Input: part model. Units: mm. Frame: model coordinates. Coordinates: 2 decimals unless noted, no trailing zeros. Order: outer loops, then holes, each group sorted by start corner. A loop starts at its lowest first (then second) coordinate and runs counter-clockwise, first axis right, second up.
Autodesk Inventor part; units mm, degrees
ref_plane "Start Plane" through (0, 0, -7.3433) normal (0, 0, 1) x (1, 0, 0)
ref_plane "End Plane" through (0, 0, 344.1675) normal (0, 0, 1) x (1, 0, 0)
ref_plane "Work Plane4" through (-6.6869, -8.3122, -7.3679) normal (0.3562, 0.4428, -0.8228) x (0.2838, -0.8903, -0.3562)
ref_plane "Start Plane" through (0, 0, -7.3433) normal (0, 0, 1) x (1, 0, 0)
ref_plane "End Plane" through (0, 0, 344.1675) normal (0, 0, 1) x (1, 0, 0)
sketch "Sketch" plane through (0, 0, 0) normal (0, 0, 1) x (1, 0, 0)
  circle A0 centre (0, 0) radius 6.9342
  circle A1 centre (0, 0) radius 10.668
  dimension "d0" = 21.336
  dimension "d1" = 3.7338
extrude "Body" add sketch "Sketch" along normal up to surface (351.5108 mm away) from surface at -7.3433
sketch "Sketch3" plane through (0, 0, 0) normal (0, 0, 1) x (1, 0, 0)
  line L0 (0, 0) -> (10, 0)
ref_plane "Work Plane3" through (0, 0, 0) normal (0, -1, 0) x (1, 0, 0)
sketch "Sketch4" plane through (0, 0, 0) normal (0, -1, 0) x (1, 0, 0)
  line L0 (-2, -7.3433) -> (12, -7.3433)
  line L1 (-2, 344.1675) -> (12, 344.1675)
  dimension "d7" = 351.5108
ref_plane "Work Plane4" through (-6.6869, -8.3122, -7.3679) normal (0.3562, 0.4428, -0.8228) x (0.2838, -0.8903, -0.3562)
split "Split1" plane through (-6.6869, -8.3122, -7.3679) removes the side toward (0.3562, 0.4428, -0.8228)
ref_plane "Work Plane5" through (6.3956, -8.5383, -22.5235) normal (-0.5418, 0.7233, -0.4281) x (0.4867, 0.6852, 0.5418)
split "Split2" plane through (6.3956, -8.5383, -22.5235) removes the side toward (-0.5418, 0.7233, -0.4281)
ref_plane "Work Plane6" through (-10.4471, 2.1596, -41.6241) normal (0.9486, -0.1961, -0.2483) x (-0.1971, 0.2475, -0.9486)
split "Split3" plane through (-10.4471, 2.1596, -41.6241) removes the side toward (0.9486, -0.1961, -0.2483)
ref_plane "Work Plane7" through (-0.5919, -10.6516, 344.93) normal (0.026, 0.467, 0.8839) x (0.9996, -0.0064, -0.026)
split "Split4" plane through (-0.5919, -10.6516, 344.93) removes the side toward (0.026, 0.467, 0.8839)
ref_plane "Work Plane8" through (-10.4471, 2.1596, 352.5336) normal (0.7628, -0.1577, 0.6272) x (0.6424, 0.0739, -0.7628)
split "Split5" plane through (-10.4471, 2.1596, 352.5336) removes the side toward (0.7628, -0.1577, 0.6272)
ref_plane "Work Plane9" through (6.3956, -8.5383, 369.7521) normal (-0.5658, 0.7554, 0.3305) x (0.7594, 0.3213, 0.5658)
split "Split6" plane through (6.3956, -8.5383, 369.7521) removes the side toward (-0.5658, 0.7554, 0.3305)
equation "\"d0\" = G_H"
equation "\"d1\" = G_T"
equation "\"d2\" = G_L"
equation "\"G_H\" = 21.336"
equation "\"G_T\" = 3.7338"
equation "\"G_L\" = 351.51084"
equation "\"G_OFFSET_START\" = 7.34335"
equation "\"G_OFFSET_END\" = 4.88279"
equation "\"d4\" = -G_OFFSET_START"
equation "\"d5\" = G_OFFSET_END + B_L"
equation "\"B_L\" = 339.28471"
properties part number "ANSI - 1/2 x 0.147 - 13.839" material "Steel, Mild"
Item 1: Draft query along X for faces 1 (the face through (5.735, -8.995, 165.952)), 2 (the face through (-0.903, -6.875, 166.412)), 3 (the face through (-6.44, 3.09, 13.37)). Return one class per face: pulls with the +X half, pulls with the -X half, needs draft (parallel to the pull), parting line crosses it, or undercut.
Response values:
face 1: parting line crosses it
face 2: undercut
face 3: pulls with the -X half
Item 2: Ray query, probe 1 along Y at (x, z) = (0, 224.5); probe 2 along X at (y, z) = (4.5, 117). Return the intervals inside material, ascending.
Response values:
probe 1: y = -10.67 to -6.93, 6.93 to 10.67
probe 2: x = -9.67 to -5.28, 5.28 to 9.67
Item 3: Cut plane C-C on z = 320. Return loops of the section in (x, y).
Response values:
outline: (-10.66, 0.46) arc R10.67 ccw (long way) to (2.56, 10.36) - (-2.79, 6.35) arc R6.93 cw (long way) to (-5.31, 4.46) - close
Item 4: Pin query (flat end, axial travel): pin 1 Ø1 at (x, y) = (7, -6.5) entering from +Z; pin 2 Ø1.5 at (y, z) = (-6.5, 48.5) entering from -X; pin 3 Ø10 at (y, z) = (-5, 270) entering from -X; pin 4 Ø8 at (x, y) = (-6.5, 3.5) entering from -Z. Return the tip coordinate at first contact, or that it passes through.
Response values:
pin 1: stops at z = 329.76
pin 2: stops at x = -8.99
pin 3: stops at x = -10.67
pin 4: stops at z = 7.94
Item 5: Cut plane B-B on z = 249. Return loops of the section in (x, y).
Response values:
outline: circle Ø21.34 at (0, 0); hole circle Ø13.87 at (0, 0)
Item 6: Cut plane A-A on y = 0. Return loops of the section in (x, z).
Response values:
outline: (-10.67, 13.5) - (-6.93, 8.77) - (-6.93, 327.42) - (-10.67, 321.02) - close; (6.93, 26.48) - (10.67, 40.75) - (10.67, 326.31) - (6.93, 330.85) - close
